from build123d import *

# Parameters (mm, degrees)
PAD003_DEPTH    = 10
SKETCH012_W     = 19
SKETCH012_H     = 10
PAD004_DEPTH    = 30
SKETCH013_R     = 1.6
POCKET006_DEPTH = 10.001
PAD005_DEPTH    = 19
SKETCH015_R     = 2.5
PAD006_DEPTH    = 10


with BuildPart() as part:
    # Sketch010 → Pad003 (new body)
    with BuildSketch(Plane.XZ):
        with BuildLine():
            Line((9.5, 0), (9.5, 70))
            ThreePointArc((9.5, 70), (6.004017, 73.968119), (1.627017, 71))
            Line((-1.627017, 71), (1.627017, 71))
            ThreePointArc((-1.627017, 71), (-6.004017, 73.968119), (-9.5, 70))
            Line((-9.5, 70), (-9.5, 0))
            Line((-9.5, 0), (9.5, 0))
        make_face()
    extrude(amount=PAD003_DEPTH)

    # Sketch012 (on Face8 of Pad003) → Pad004 (join)
    with BuildSketch(Plane.XZ.offset(10)):
        with Locations((0, 5)):
            Rectangle(SKETCH012_W, SKETCH012_H)
    extrude(amount=PAD004_DEPTH)

    # Sketch013 (on Face6 of Pad004) → Pocket006 (cut, through all)
    with BuildSketch(Plane(origin=(0, 0, 10), x_dir=(-1, 0, 0), z_dir=(0, 0, 1))):
        with Locations((-4, 25)):
            Circle(SKETCH013_R)
        with Locations((4, 35)):
            Circle(SKETCH013_R)
    extrude(amount=-POCKET006_DEPTH, mode=Mode.SUBTRACT)

    # Sketch014 (on Face10 of Pocket006) → Pad005 (join)
    with BuildSketch(Plane(origin=(9.5, 0, 0), x_dir=(0, 0, 1), z_dir=(1, 0, 0))):
        Polygon((10, 17.517339), (17.517341, 10), (10, 10), align=None)
    extrude(amount=-PAD005_DEPTH)

    # Sketch015 (on Face4 of Pad005) → Pad006 (join)
    with BuildSketch(Plane.XZ.offset(10)):
        with Locations((-5.5, 70)):
            Circle(SKETCH015_R)
        with Locations((5.5, 70)):
            Circle(SKETCH015_R)
    extrude(amount=PAD006_DEPTH)


solid = part.part
Geometry: final body of the model. Coordinates: model frame, mm. A direction names the side the tool comes from. Give positions to 0.01 mm unless a question says otherwise; leave off trailing zeros. Loops run counter-clockwise (first coordinate to the right, second up) from the corner with the lowest first, then second, coordinate; pieces in that order, holes last. Notation, with made-up numbers: (10, -6.5) -> (29, -6.5) arc R23 ccw to (29, 17.5) -> close; hole circle Ø8 at (78.5, 64.25). An arc over 180 degrees is marked (long way). Put each result on its own line as item: value.
1. Pull-direction query (X, two-part tool) for faces 4 (the flat face through (-9.5, -9.7, 22.2)), 5 (the flat face through (0, -20, 0)), 6 (the cylindrical face through (-4.74, -33.58, 5.07)); classes: released by +X, released by -X, zero draft, split by the parting line, or undercut.
Taken from the geometry:
face 4: released by -X
face 5: zero draft
face 6: undercut
2. Cut plane B-B (x = 4). Return the cut outline in (y, z).
Taken from the geometry:
outline: (-40, 0) -> (-26.6, 0) -> (-26.6, 10) -> (-40, 10) -> close; (-23.4, 0) -> (0, 0) -> (0, 73.71) -> (-10, 73.71) -> (-10, 72) -> (-20, 72) -> (-20, 68) -> (-10, 68) -> (-10, 17.52) -> (-17.52, 10) -> (-23.4, 10) -> close
3. Pin query (flat end, axial travel): P1, Ø1, axis at x = -2.5, z = 54.5, coming from the -Y side; P2, Ø2.5, axis at x = 4, y = -25, coming from the +Z side; P3, Ø9.5, axis at x = 4.5, y = -27, coming from the +Z side; P4, Ø10, axis at x = -2.5, y = -28.5, coming from the -Z side. Return the tip coordinate at first contact, or that it passes through.
Taken from the geometry:
P1: stops at y = -10
P2: passes through
P3: stops at z = 10
P4: stops at z = 0
4. Set-up query: faces 1 (the flat face through (0.13, -13.81, 13.71)), 2 (the cylindrical face through (7, -15, 68)), 3 (the flat face through (-6, -20, 70)). Return all of +Z, -Z, +X, -X, +Y, -Y with unobstructed straight access to the full face (end or side cutting, diameter ignored); none if empty.
Taken from the geometry:
face 1: +X, -X, -Y
face 2: -Y
face 3: +Z, +X, -X, -Y
5. Cut plane C-C (y = -8.5). Return the cut outline in (x, z), plus the area to 3 significant figures.
Taken from the geometry:
outline: (-9.5, 0) -> (9.5, 0) -> (9.5, 70) arc R4 ccw to (1.63, 71) -> (-1.63, 71) arc R4 ccw to (-9.5, 70) -> close
area: 1,380 mm2
6. Cut plane D-D (z = 35). Return the cut outline in (x, y), plus the area to 3 significant figures.
Taken from the geometry:
outline: (-9.5, -10) -> (9.5, -10) -> (9.5, 0) -> (-9.5, 0) -> close
area: 190 mm2
7. Cut plane A-A (y = -35). Return the cut outline in (x, z), plus the area to 3 significant figures.
Taken from the geometry:
outline: (-9.5, 0) -> (-5.6, 0) -> (-5.6, 10) -> (-9.5, 10) -> close; (-2.4, 0) -> (9.5, 0) -> (9.5, 10) -> (-2.4, 10) -> close
area: 158 mm2
8. Ray query, line 1 along X through (y, z) = (-35, 4); line 2 along Y through (x, z) = (4, 3); line 3 along Y through (x, z) = (-4, 7.75). Return the intervals inside material, ascending. Write a range as [from, to].
Taken from the geometry:
line 1: x = [-9.5, -5.6], [-2.4, 9.5]
line 2: y = [-40, -26.6], [-23.4, 0]
line 3: y = [-40, -36.6], [-33.4, 0]
